Check sheet for the modelled part. Datum: model origin and axes. Units: mm. Face numbers are marked on the shaded views. A direction names the side the tool comes from. Give positions to 0.01 mm unless a question says otherwise; leave off trailing zeros. Write each loop counter-clockwise with the first axis right and the second up, starting at its lowest first coordinate (ties: lowest second). Pieces come first, ordered by that corner, then holes. Notation, with made-up numbers: (77.25, 48.5) -> (127.25, 48.5) arc R16 ccw to (127.25, 76.5) -> close; hole circle Ø5 at (8.5, -5). An arc over 180 degrees is marked (long way). Return JSON: item names as keys, results as strings.
from build123d import *

# Parameters (mm, degrees)
SKETCH1_W           = 97.46
SKETCH1_H           = 97.46
BOSS_EXTRUDE1_DEPTH = 1.27
SKETCH3_W           = 5
SKETCH3_H           = 97.46
BOSS_EXTRUDE2_DEPTH = 3.73
SKETCH7_R           = 1
CUT_EXTRUDE2_DEPTH  = 5
SKETCH6_R           = 1
CUT_EXTRUDE3_DEPTH  = 5
SKETCH4_R           = 1
CUT_EXTRUDE4_DEPTH  = 5
SKETCH5_R           = 1
CUT_EXTRUDE5_DEPTH  = 5
CUT_EXTRUDE7_REACH  = 99.46
SKETCH10_R          = 1
CUT_EXTRUDE8_REACH  = 99.46
SKETCH9_R           = 1
CUT_EXTRUDE9_DEPTH  = 1.27
CUT_EXTRUDE10_DEPTH = 1.27
SKETCH13_W          = 87.46
SKETCH13_H          = 94.92
BOSS_EXTRUDE3_DEPTH = 1.27
SKETCH8_R           = 1.4
CUT_EXTRUDE6_DEPTH  = 10


with BuildPart() as part:
    # Sketch1 → Boss-Extrude1 (new body)
    with BuildSketch(Plane.XY):
        with Locations((48.73, 48.73)):
            Rectangle(SKETCH1_W, SKETCH1_H)
    extrude(amount=BOSS_EXTRUDE1_DEPTH)

    # Sketch3 → Boss-Extrude2 (add)
    with BuildSketch(Plane.XY.offset(1.27)):
        with Locations((2.5, 48.73)):
            Rectangle(SKETCH3_W, SKETCH3_H)
        with Locations((94.96, 48.73)):
            Rectangle(SKETCH3_W, SKETCH3_H)
    extrude(amount=BOSS_EXTRUDE2_DEPTH)

    # Sketch7 → Cut-Extrude2 (cut)
    with BuildSketch(Plane(origin=(0, 97.46, 0), x_dir=(-1, 0, 0), z_dir=(0, 1, 0))):
        with Locations((-2.5, 2.5)):
            Circle(SKETCH7_R)
    extrude(amount=-CUT_EXTRUDE2_DEPTH, mode=Mode.SUBTRACT)

    # Sketch6 → Cut-Extrude3 (cut)
    with BuildSketch(Plane(origin=(0, 97.46, 0), x_dir=(-1, 0, 0), z_dir=(0, 1, 0))):
        with Locations((-94.96, 2.5)):
            Circle(SKETCH6_R)
    extrude(amount=-CUT_EXTRUDE3_DEPTH, mode=Mode.SUBTRACT)

    # Sketch4 → Cut-Extrude4 (cut)
    with BuildSketch(Plane.XZ):
        with Locations((94.96, 2.5)):
            Circle(SKETCH4_R)
    extrude(amount=-CUT_EXTRUDE4_DEPTH, mode=Mode.SUBTRACT)

    # Sketch5 → Cut-Extrude5 (cut)
    with BuildSketch(Plane.XZ):
        with Locations((2.5, 2.5)):
            Circle(SKETCH5_R)
    extrude(amount=-CUT_EXTRUDE5_DEPTH, mode=Mode.SUBTRACT)

    # Sketch10 → Cut-Extrude7 (cut, up to next)
    with BuildSketch(Plane.ZY, mode=Mode.PRIVATE) as cut_extrude7_sk1:
        with Locations((2.5, 23.73)):
            Circle(SKETCH10_R)
    cut_extrude7_tool1 = extrude(cut_extrude7_sk1.sketch, amount=-CUT_EXTRUDE7_REACH, mode=Mode.PRIVATE) & part.part
    add(cut_extrude7_tool1.solids().sort_by_distance((0, 23.73, 2.5))[0], mode=Mode.SUBTRACT)
    # Sketch10 → Cut-Extrude7 (cut, up to next)
    with BuildSketch(Plane.ZY, mode=Mode.PRIVATE) as cut_extrude7_sk2:
        with Locations((2.5, 73.73)):
            Circle(SKETCH10_R)
    cut_extrude7_tool2 = extrude(cut_extrude7_sk2.sketch, amount=-CUT_EXTRUDE7_REACH, mode=Mode.PRIVATE) & part.part
    add(cut_extrude7_tool2.solids().sort_by_distance((0, 73.73, 2.5))[0], mode=Mode.SUBTRACT)

    # Sketch9 → Cut-Extrude8 (cut, up to next)
    with BuildSketch(Plane(origin=(97.46, 0, 0), x_dir=(0, 0, -1), z_dir=(1, 0, 0)), mode=Mode.PRIVATE) as cut_extrude8_sk1:
        with Locations((-2.5, 73.73)):
            Circle(SKETCH9_R)
    cut_extrude8_tool1 = extrude(cut_extrude8_sk1.sketch, amount=-CUT_EXTRUDE8_REACH, mode=Mode.PRIVATE) & part.part
    add(cut_extrude8_tool1.solids().sort_by_distance((97.46, 73.73, 2.5))[0], mode=Mode.SUBTRACT)
    # Sketch9 → Cut-Extrude8 (cut, up to next)
    with BuildSketch(Plane(origin=(97.46, 0, 0), x_dir=(0, 0, -1), z_dir=(1, 0, 0)), mode=Mode.PRIVATE) as cut_extrude8_sk2:
        with Locations((-2.5, 23.73)):
            Circle(SKETCH9_R)
    cut_extrude8_tool2 = extrude(cut_extrude8_sk2.sketch, amount=-CUT_EXTRUDE8_REACH, mode=Mode.PRIVATE) & part.part
    add(cut_extrude8_tool2.solids().sort_by_distance((97.46, 23.73, 2.5))[0], mode=Mode.SUBTRACT)

    # Sketch11 → Cut-Extrude9 (cut)
    with BuildSketch(Plane(origin=(0, 0, 0), x_dir=(-1, 0, 0), z_dir=(0, -1, 0))):
        Polygon((-92.46, -5), (-97.46, -5), (-97.46, 0), (0, 0), (0, -5), (-5, -5), (-5, -1.27), (-92.46, -1.27), align=None)
    extrude(amount=-CUT_EXTRUDE9_DEPTH, mode=Mode.SUBTRACT)

    # Sketch12 → Cut-Extrude10 (cut)
    with BuildSketch(Plane(origin=(0, 97.46, 0), x_dir=(1, 0, 0), z_dir=(0, 1, 0))):
        Polygon((92.46, -1.27), (92.46, -5), (97.46, -5), (97.46, 0), (0, 0), (0, -5), (5, -5), (5, -1.27), align=None)
    extrude(amount=-CUT_EXTRUDE10_DEPTH, mode=Mode.SUBTRACT)

    # Sketch13 → Boss-Extrude3 (add)
    with BuildSketch(Plane.XY.offset(1.27)):
        with Locations((48.73, 48.73)):
            Rectangle(SKETCH13_W, SKETCH13_H)
    extrude(amount=BOSS_EXTRUDE3_DEPTH)

    # Sketch8 → Cut-Extrude6 (cut)
    with BuildSketch(Plane(origin=(0, 0, 0), x_dir=(-1, 0, 0), z_dir=(0, 0, -1))):
        with Locations((-31.864061653, 37.943406611)):
            Circle(SKETCH8_R)
        with Locations((-89.874061653, 86.953406611)):
            Circle(SKETCH8_R)
        with Locations((-31.864061653, 86.953406611)):
            Circle(SKETCH8_R)
        with Locations((-89.874061653, 37.943406611)):
            Circle(SKETCH8_R)
    extrude(amount=-CUT_EXTRUDE6_DEPTH, mode=Mode.SUBTRACT)


solid = part.part
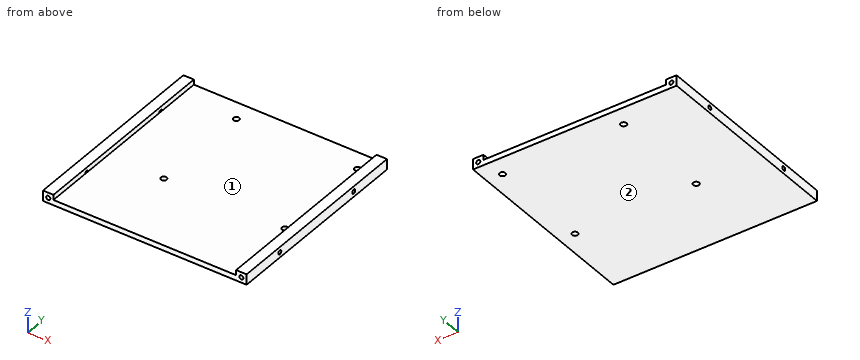
(1) Depth check by flat-ended pin: pin 1 Ø0.8 at (y, z) = (74, 2) entering from -X; pin 2 Ø2 at (x, y) = (31.86, 37.94) entering from -Z; pin 3 Ø0.6 at (x, z) = (95, 2.5) entering from +Y; pin 4 Ø0.8 at (y, z) = (23.5, 2) entering from +X. Enter the tip coordinate at first touch or a pass-through.
Reply:
{"pin 1": "x = 5", "pin 2": "through", "pin 3": "y = 92.46", "pin 4": "x = 92.46"}
(2) Set-up check for the marked faces 1 and 2: record each of +Z, -Z, +X, -X, +Y, -Y from which the full face is reachable in a straight line by a thin tool's end or side.
Reply:
{"face 1": "+Z, +Y, -Y", "face 2": "-Z, +X, -X, +Y, -Y"}
(3) Cross-section at B-B on y = 43.5. Enter the section's corners in (x, z), then the cut area to 3 significant figures.
Reply:
{"outline": "(0, 0) -> (97.46, 0) -> (97.46, 5) -> (92.46, 5) -> (92.46, 2.54) -> (5, 2.54) -> (5, 5) -> (0, 5) -> close", "area": "272 mm^2"}
(4) Cross-section at C-C on x = 25. Enter the section's corners in (y, z).
Reply:
{"outline": "(1.27, 0) -> (96.19, 0) -> (96.19, 2.54) -> (1.27, 2.54) -> close"}
(5) Thickness scan on L1, parallel to Y at x = 1.1, z = 2.5; L2, parallel to X at y = 21, z = 3.6; L3, parallel to Z at x = 3.6, y = 73.73. Record the ranges inside material, lowest first.
Reply:
{"L1": "1.27 to 22.73, 24.73 to 72.73, 74.73 to 96.19", "L2": "0 to 5, 92.46 to 97.46", "L3": "0 to 1.5, 3.5 to 5"}
(6) Cross-section at A-A on z = 4.25. Enter the section's corners in (x, y).
Reply:
{"outline": "(0, 1.27) -> (5, 1.27) -> (5, 96.19) -> (0, 96.19) -> close; (92.46, 1.27) -> (97.46, 1.27) -> (97.46, 96.19) -> (92.46, 96.19) -> close"}
